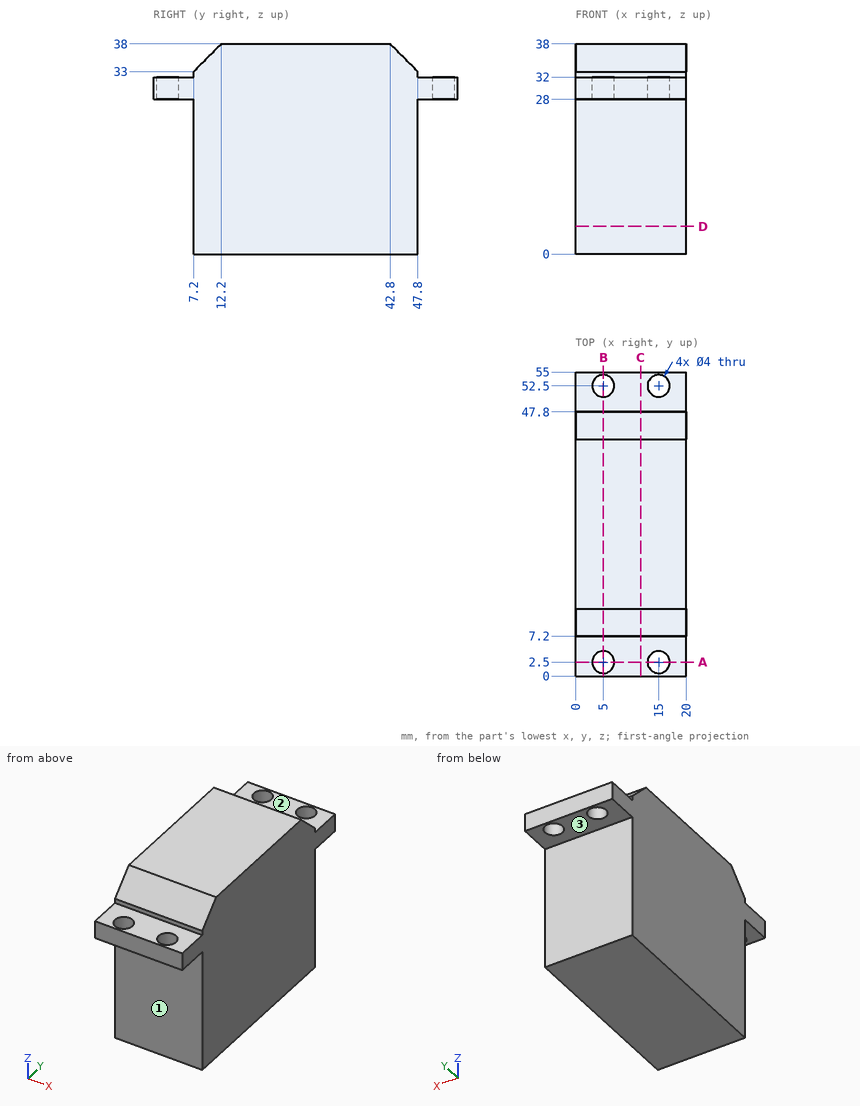
Answer from the drawing. Dimensions are ordinates in mm from the lowest x, y and z of the part. A direction names the side the tool comes from. Give positions to 0.01 mm unless a question says otherwise; leave off trailing zeros. Write each loop counter-clockwise with the first axis right and the second up, starting at its lowest first coordinate (ties: lowest second). Pieces come first, ordered by that corner, then holes. Notation, with made-up numbers: (89.5, 29.25) -> (125.5, 29.25) arc R27 ccw to (125.5, 52.25) -> close; hole circle Ø3 at (-38, 57). An arc over 180 degrees is marked (long way). Use a Markdown table: item, result.
(1) Section D-D, the plane z = 5 is taken. Determine the outline of the cut face in (x, y), then the cut area to 3 significant figures.
Return value:
| item | result |
|---|---|
| outline | (0, 7.2) -> (20, 7.2) -> (20, 47.8) -> (0, 47.8) -> close |
| area | 812 mm2 |
(2) Section C-C, the plane x = 11.75 is taken. Determine the outline of the cut face in (y, z), then the cut area to 3 significant figures.
Return value:
| item | result |
|---|---|
| outline | (0, 28) -> (7.2, 28) -> (7.2, 0) -> (47.8, 0) -> (47.8, 28) -> (55, 28) -> (55, 32) -> (47.8, 32) -> (47.8, 33) -> (42.8, 38) -> (12.2, 38) -> (7.2, 33) -> (7.2, 32) -> (0, 32) -> close |
| area | 1,580 mm2 |
(3) For the marked faces 1, 2 and 3, determine the directions among +Z, -Z, +X, -X, +Y, -Y from which every point of the face is accessible in a straight line to the end or side of a thin tool.
Return value:
| item | result |
|---|---|
| face 1 | -Z, +X, -X, -Y |
| face 2 | +Z, +X, -X, +Y |
| face 3 | -Z, +X, -X, +Y |
(4) Flat-ended cylindrical pins translate along their axes: P1, Ø6.5, axis at x = 15, y = 52.5, coming from the -Z side; P2, Ø6, axis at x = 6.5, z = 10, coming from the +Y side; P3, Ø4.5, axis at x = 5, y = 2.5, coming from the +Z side; P4, Ø3, axis at x = 5, y = 52.5, coming from the -Z side. Find the tip coordinate at first contact, or state that the pin passes through.
Return value:
| item | result |
|---|---|
| P1 | z = 28 |
| P2 | y = 47.8 |
| P3 | z = 32 |
| P4 | through |
(5) Section B-B, the plane x = 5 is taken. Determine the outline of the cut face in (y, z), then the cut area to 3 significant figures.
Return value:
| item | result |
|---|---|
| outline | (0, 28) -> (0.5, 28) -> (0.5, 32) -> (0, 32) -> close; (4.5, 28) -> (7.2, 28) -> (7.2, 0) -> (47.8, 0) -> (47.8, 28) -> (50.5, 28) -> (50.5, 32) -> (47.8, 32) -> (47.8, 33) -> (42.8, 38) -> (12.2, 38) -> (7.2, 33) -> (7.2, 32) -> (4.5, 32) -> close; (54.5, 28) -> (55, 28) -> (55, 32) -> (54.5, 32) -> close |
| area | 1,540 mm2 |
(6) Find the intervals of material crossed by probe 1 along Y at (x, z) = (15, 29.5); probe 2 along X at (y, z) = (52.5, 29.1); probe 3 along X at (y, z) = (52, 29), in increasing order. Write a range as from..to.
Return value:
| item | result |
|---|---|
| probe 1 | 0..0.5, 4.5..50.5, 54.5..55 |
| probe 2 | 0..3, 7..13, 17..20 |
| probe 3 | 0..3.06, 6.94..13.06, 16.94..20 |
(7) Section A-A, the plane y = 2.5 is taken. Determine the outline of the cut face in (x, z), then the cut area to 3 significant figures.
Return value:
| item | result |
|---|---|
| outline | (0, 28) -> (3, 28) -> (3, 32) -> (0, 32) -> close; (7, 28) -> (13, 28) -> (13, 32) -> (7, 32) -> close; (17, 28) -> (20, 28) -> (20, 32) -> (17, 32) -> close |
| area | 48.0 mm2 |
